from build123d import *

# Parameters (mm, degrees)
SKETCH1_R           = 2.4892
SKETCH1_R_2         = 12.3825
SKETCH1_R_3         = 14.3002
SKETCH1_R_4         = 11.1252
SKETCH1_R_5         = 40.3225
BOSS_EXTRUDE1_DEPTH = 6.35
FILLET2_R           = 6.35


with BuildPart() as part:
    # Sketch1 → Boss-Extrude1 (new body)
    with BuildSketch(Plane(origin=(0, 0, 0), x_dir=(1, 0, 0), z_dir=(0, 1, 0))):
        with BuildLine():
            ThreePointArc((-173.478687828, 72.590962089), (-186.178687828, 59.890962089), (-173.478687828, 47.190962089))
            Line((-173.478687828, 47.190962089), (-150.271339409, 45.094655518))
            Line((-150.271339409, 45.094655518), (-98.200516404, -45.094655518))
            Line((-98.200516404, -45.094655518), (-110.67256166, -48.892439461))
            ThreePointArc((-110.67256166, -48.892439461), (-116.589819654, -63.177963961), (-104.32256166, -72.590962089))
            Line((-104.32256166, -72.590962089), (104.322561739, -72.590962089))
            ThreePointArc((104.322561739, -72.590962089), (116.589819664, -63.177963923), (110.67256166, -48.892439461))
            Line((110.67256166, -48.892439461), (98.200516404, -45.094655518))
            Line((98.200516404, -45.094655518), (150.271339409, 45.094655518))
            Line((150.271339409, 45.094655518), (173.478687828, 47.190962089))
            ThreePointArc((173.478687828, 47.190962089), (186.178687828, 59.890962094), (173.478687816, 72.590962089))
            Line((173.478687816, 72.590962089), (-173.478687828, 72.590962089))
        make_face()
        with Locations(Location((173.478687828, 59.890962089, 0), (0, 0, 270))):
            Circle(SKETCH1_R, mode=Mode.SUBTRACT)
        with Locations(Location((-104.32256166, -59.890962089, 0), (0, 0, 270))):
            Circle(SKETCH1_R, mode=Mode.SUBTRACT)
        with Locations(Location((-67.13289048, -59.890962089, 0), (0, 0, 270))):
            Circle(SKETCH1_R, mode=Mode.SUBTRACT)
        with Locations(Location((-67.13289048, -34.490962089, 0), (0, 0, 270))):
            Circle(SKETCH1_R_2, mode=Mode.SUBTRACT)
        with Locations(Location((-67.13289048, -9.090962089, 0), (0, 0, 270))):
            Circle(SKETCH1_R, mode=Mode.SUBTRACT)
        with Locations(Location((15.87430952, -34.490962089, 0), (0, 0, 270))):
            Circle(SKETCH1_R_3, mode=Mode.SUBTRACT)
        with Locations(Location((81.671791392, -43.565397329, 0), (0, 0, 270))):
            Circle(SKETCH1_R, mode=Mode.SUBTRACT)
        with Locations(Location((-26.911726221, -28.671379147, 0), (0, 0, 270))):
            Circle(SKETCH1_R_4, mode=Mode.SUBTRACT)
        with Locations(Location((-173.478687828, 59.890962089, 0), (0, 0, 270))):
            Circle(SKETCH1_R, mode=Mode.SUBTRACT)
        with Locations(Location((72.644027153, 3.985206637, 0), (0, 0, 270))):
            Circle(SKETCH1_R_5, mode=Mode.SUBTRACT)
        with Locations(Location((35.710881273, 46.848232392, 0), (0, 0, 270))):
            Circle(SKETCH1_R, mode=Mode.SUBTRACT)
        with Locations(Location((91.297923401, 57.401762089, 0), (0, 0, 270))):
            Circle(SKETCH1_R, mode=Mode.SUBTRACT)
        with Locations(Location((104.32256166, -59.890962089, 0), (0, 0, 270))):
            Circle(SKETCH1_R, mode=Mode.SUBTRACT)
    extrude(amount=BOSS_EXTRUDE1_DEPTH)

    # Fillet2
    fillet2_edges = [part.edges().sort_by_distance(p)[0] for p in [
        (150.271339409, 3.175, -45.094655518),
        (98.200516404, 3.175, 45.094655518),
        (-98.200516404, 3.175, 45.094655518),
        (-150.271339409, 3.175, -45.094655518),
    ]]
    fillet(fillet2_edges, radius=FILLET2_R)


solid = part.part
The listing builds one solid part. Answer for the finished solid, in the listing's coordinates (mm). A direction names the side the tool comes from. Give positions to 0.01 mm unless a question says otherwise; leave off trailing zeros. Write each loop counter-clockwise with the first axis right and the second up, starting at its lowest first coordinate (ties: lowest second). Pieces come first, ordered by that corner, then holes. Notation, with made-up numbers: (49.5, -12) -> (79.5, -12) arc R31 cw to (79.5, 14) -> close; hole circle Ø3 at (-15.75, 27). An arc over 180 degrees is marked (long way). One line per question, with ' | ' between items. Start each with the question number.
1. Section B-B (z = -28.5) is taken. Determine the outline of the cut face in (x, y).
2. Section C-C (y = 1) is taken. State how many separate pieces and enclosed holes the cut face has, plus the area to 3 significant figures.
3. Given pin 1 Ø8 at (x, z) = (-50.5, 32) entering from -Y; pin 2 Ø1 at (y, z) = (2.5, -15.5) entering from +X, each flat-ended and moving along its own axis, determine where each tip first touches the part or whether it passes through.
4. Section A-A (z = 33) is taken. Determine the outline of the cut face in (x, y), plus the area to 3 significant figures.
5. Find the intervals of material crossed by probe 1 along X at (y, z) = (2, 27); probe 2 along X at (y, z) = (1.25, 32.5); probe 3 along X at (y, z) = (2, 38), in increasing order.
6. Section D-D (x = 143) is taken. Determine the outline of the cut face in (y, z), plus the area to 3 significant figures.
7. For faces 4 (the cylindrical face through (-36.782, 3.131, 33.805)), 5 (the flat face through (125.1, 3.1, -1.5)), 6 (the flat face through (-125.735, 3.131, -2.597)), determine the directions among +Z, -Z, +X, -X, +Y, -Y from which every point of the face is accessible in a straight line to the end or side of a thin tool.
8. For a pull along X with two mould halves and no side action, classify faces 1 (the cylindrical face through (33.28, 3.13, -12.73)), 2 (the flat face through (-3, 6.35, -17)), 3 (the cylindrical face through (-116.65, 3.13, 62.95)) as pulls with the +X half, pulls with the -X half, needs draft (parallel to the pull), parting line crosses it, or undercut.
Response values:
1) outline: (-140.69, 0) -> (40.63, 0) -> (40.63, 6.35) -> (-140.69, 6.35) -> close; (104.66, 0) -> (140.69, 0) -> (140.69, 6.35) -> (104.66, 6.35) -> close
2) separate pieces: 1 | enclosed holes: 13 | area: 31,900 mm2
3) pin 1: y = 0 | pin 2: x = 133.47
4) outline: (-105.18, 0) -> (-79.43, 0) -> (-79.43, 6.35) -> (-105.18, 6.35) -> close; (-54.84, 0) -> (-37.16, 0) -> (-37.16, 6.35) -> (-54.84, 6.35) -> close; (-16.66, 0) -> (1.65, 0) -> (1.65, 6.35) -> (-16.66, 6.35) -> close; (30.1, 0) -> (56.58, 0) -> (56.58, 6.35) -> (30.1, 6.35) -> close; (88.71, 0) -> (105.18, 0) -> (105.18, 6.35) -> (88.71, 6.35) -> close | area: 665 mm2
5) probe 1: -108.65 to -76.99, -57.27 to -37.91, -15.91 to 3.69, 28.06 to 46.84, 98.45 to 108.65 | probe 2: -105.47 to -79.35, -54.91 to -37.36, -16.47 to 1.71, 30.04 to 55.48, 89.81 to 105.47 | probe 3: -102.3 to -79.01, -55.26 to -32.97, -20.85 to 2.01, 29.74 to 102.3
6) outline: (0, -72.59) -> (6.35, -72.59) -> (6.35, -32.5) -> (0, -32.5) -> close | area: 255 mm2
7) face 4: +Y, -Y | face 5: +X, +Y, -Y | face 6: -X, +Y, -Y
8) face 1: undercut | face 2: needs draft | face 3: pulls with the -X half
